from build123d import *

# Parameters (mm, degrees)
BOSS_EXTRUDE1_DEPTH = 3
SKETCH2_W           = 54
SKETCH2_H           = 8
BOSS_EXTRUDE2_DEPTH = 57
SKETCH3_R           = 2.05
CUT_EXTRUDE1_DEPTH  = 57
BOSS_EXTRUDE3_DEPTH = 57
FILLET1_R           = 3
CUT_EXTRUDE2_DEPTH  = 6
FILLET2_R           = 1
FILLET3_R           = 0.8
CHAMFER1_SIZE       = 0.8
CHAMFER2_SIZE       = 0.7


with BuildPart() as part:
    # Sketch1 → Boss-Extrude1 (new body)
    with BuildSketch(Plane.XY):
        Polygon((54, 0), (54, 8), (30, 8), (30, 38), (0, 38), (0, 0), align=None)
    extrude(amount=BOSS_EXTRUDE1_DEPTH)

    # Sketch2 → Boss-Extrude2 (add)
    with BuildSketch(Plane(origin=(0, 0, 0), x_dir=(-1, 0, 0), z_dir=(0, 0, -1))):
        with Locations((-27, 4)):
            Rectangle(SKETCH2_W, SKETCH2_H)
    extrude(amount=BOSS_EXTRUDE2_DEPTH)

    # Sketch3 → Cut-Extrude1 (cut)
    with BuildSketch(Plane.XZ):
        with Locations(Location((40, -1.8, 0), (0, 0, 270))):
            Circle(SKETCH3_R)
        with Locations(Location((40, -50.3, 0), (0, 0, 270))):
            Circle(SKETCH3_R)
    extrude(amount=-CUT_EXTRUDE1_DEPTH, mode=Mode.SUBTRACT)

    # Sketch4 → Boss-Extrude3 (add)
    with BuildSketch(Plane(origin=(0, 0, 0), x_dir=(-1, 0, 0), z_dir=(0, 0, -1))):
        Polygon((-18, 8), (-18, 11), (-23, 11), (-23, 12.85), (-18.25, 17.6), (-11.75, 17.6), (-7, 12.85), (-7, 11), (-12, 11), (-12, 8), align=None)
    extrude(amount=BOSS_EXTRUDE3_DEPTH)

    # Fillet1
    fillet1_edges = [part.edges().sort_by_distance(p)[0] for p in [
        (0, 38, 1.5),
        (30, 38, 1.5),
    ]]
    fillet(fillet1_edges, radius=FILLET1_R)

    # Sketch5 → Cut-Extrude2 (cut)
    with BuildSketch(Plane.XY.offset(3)):
        with BuildLine():
            Line((27.915844453, 26.05), (30, 26.05))
            Line((30, 26.05), (30, 19.95))
            Line((30, 19.95), (27.915844453, 19.95))
            ThreePointArc((27.915844453, 19.95), (27.100066936, 19.836954631), (26.345769332, 19.506338028))
            ThreePointArc((26.345769332, 19.506338028), (20.1, 23), (26.345769332, 26.493661972))
            ThreePointArc((26.345769332, 26.493661972), (27.100066936, 26.163045369), (27.915844453, 26.05))
        make_face()
    extrude(amount=-CUT_EXTRUDE2_DEPTH, mode=Mode.SUBTRACT)

    # Fillet2
    fillet2_edges = [part.edges().sort_by_distance(p)[0] for p in [
        (30, 26.05, 1.5),
        (30, 19.95, 1.5),
        (28.957922227, 26.05, 3),
        (27.100066936, 26.163045369, 3),
        (20.1, 23, 3),
        (27.100066936, 19.836954631, 3),
        (28.957922227, 19.95, 3),
    ]]
    fillet(fillet2_edges, radius=FILLET2_R)

    # Fillet3
    fillet3_edges = [part.edges().sort_by_distance(p)[0] for p in [
        (7, 11, -28.5),
        (7, 12.85, -28.5),
        (11.75, 17.6, -28.5),
        (18.25, 17.6, -28.5),
        (23, 12.85, -28.5),
        (23, 11, -28.5),
    ]]
    fillet(fillet3_edges, radius=FILLET3_R)

    # Chamfer1
    chamfer1_edges = [part.edges().sort_by_distance(p)[0] for p in [
        (20.1, 11, -57),
        (23, 12.159314575, -57),
        (7, 12.159314575, -57),
        (9.375, 15.225, -57),
        (15, 17.6, -57),
        (20.625, 15.225, -57),
        (22.939103626, 12.824775896, -57),
        (18.224775896, 17.539103626, -57),
        (11.775224104, 17.539103626, -57),
        (7.060896374, 12.824775896, -57),
        (7.234314575, 11.234314575, -57),
        (22.765685425, 11.234314575, -57),
        (12, 9.5, -57),
        (9.9, 11, -57),
        (18, 9.5, -57),
    ]]
    chamfer(chamfer1_edges, length=CHAMFER1_SIZE)

    # Chamfer2
    chamfer2_edges = [part.edges().sort_by_distance(p)[0] for p in [
        (40, 8, -48.25),
        (40, 0, -48.25),
        (40, 8, 0.25),
        (40, 0, 0.25),
    ]]
    chamfer(chamfer2_edges, length=CHAMFER2_SIZE)


solid = part.part
Read the model definition and answer for the solid it produces. Units are mm, in the model's axes. A direction names the side the tool comes from. Give positions to 0.01 mm unless a question says otherwise; leave off trailing zeros. Loops run counter-clockwise (first coordinate to the right, second up) from the corner with the lowest first, then second, coordinate; pieces in that order, holes last. Notation, with made-up numbers: (76, 79) -> (127, 79) arc R11 ccw to (127, 83) -> close; hole circle Ø2 at (15, -18). An arc over 180 degrees is marked (long way). Use a Markdown table: item, result.
Q1. Each of these flat-tipped pins is pushed along its axis until it touches: pin 1 (0.6 mm diameter, centred on y = 12, z = -27.5, fed in from +X); pin 2 (1.8 mm diameter, centred on x = 14, z = -36.5, fed in from +Y); pin 3 (0.6 mm diameter, centred on y = 12.5, z = -38.5, fed in from -X). Where does it stop, or does it pass through?
Solved:
| item | result |
|---|---|
| pin 1 | stops at x = 23 |
| pin 2 | stops at y = 17.6 |
| pin 3 | stops at x = 7 |
Q2. Section B-B, the plane z = -1.8 is taken. Determine the outline of the cut face in (x, y), then the cut area to 3 significant figures.
Solved:
| item | result |
|---|---|
| outline | (0, 0) -> (37.25, 0) -> (37.95, 0.7) -> (37.95, 7.3) -> (37.25, 8) -> (18, 8) -> (18, 11) -> (22.2, 11) arc R0.8 ccw to (23, 11.8) -> (23, 12.52) arc R0.8 ccw to (22.77, 13.08) -> (18.48, 17.37) arc R0.8 ccw to (17.92, 17.6) -> (12.08, 17.6) arc R0.8 ccw to (11.52, 17.37) -> (7.23, 13.08) arc R0.8 ccw to (7, 12.52) -> (7, 11.8) arc R0.8 ccw to (7.8, 11) -> (12, 11) -> (12, 8) -> (0, 8) -> close; (42.05, 0.7) -> (42.75, 0) -> (54, 0) -> (54, 8) -> (42.75, 8) -> (42.05, 7.3) -> close |
| area | 499 mm^2 |
Q3. Find the intervals of material crossed by line 1 along Y through (x, z) = (11.5, -52.5); line 2 along X through (y, z) = (9.5, -46.5); line 3 along Y through (x, z) = (19, -42), in increasing order.
Solved:
| item | result |
|---|---|
| line 1 | y = 0 to 8, 11 to 17.35 |
| line 2 | x = 12 to 18 |
| line 3 | y = 0 to 8, 11 to 16.85 |
Q4. Determine the mould class of faces 1 (the face through (27, 5, -57)), 2 (the face through (12, 10, -28)), 3 (the face through (20.368, 14.908, -56.606)) for opening direction Y: pulls with the +Y half, pulls with the -Y half, needs draft (parallel to the pull), parting line crosses it, or undercut.
Solved:
| item | result |
|---|---|
| face 1 | needs draft |
| face 2 | undercut |
| face 3 | pulls with the +Y half |
Q5. A tool of negligible diameter and unlimited length cuts with its end or side. For faces 4 (the face through (18, 9, -28)), 5 (the face through (20.65, 15.2, -27.71)), 6 (the face through (15, 17.6, -28)), 7 (the face through (30, 31, 1)), 8 (the face through (6, 8, -28)), from which of +Z, -Z, +X, -X, +Y, -Y can it reach the whole face along a straight path? Write none if from no direction.
Solved:
| item | result |
|---|---|
| face 4 | -Z, +X |
| face 5 | -Z, +X, +Y |
| face 6 | -Z, +X, -X, +Y |
| face 7 | +Z, -Z, +X, +Y |
| face 8 | -Z, -X |
Q6. Section A-A, the plane x = 40 is taken. Determine the outline of the cut face in (y, z).
Solved:
| item | result |
|---|---|
| outline | (0, -57) -> (8, -57) -> (8, -53.05) -> (7.3, -52.35) -> (0.7, -52.35) -> (0, -53.05) -> close; (0, -47.55) -> (0.7, -48.25) -> (7.3, -48.25) -> (8, -47.55) -> (8, -4.55) -> (7.3, -3.85) -> (0.7, -3.85) -> (0, -4.55) -> close; (0, 0.95) -> (0.7, 0.25) -> (7.3, 0.25) -> (8, 0.95) -> (8, 3) -> (0, 3) -> close |
Q7. Section D-D, the plane z = -25.5 is taken. Determine the outline of the cut face in (x, y).
Solved:
| item | result |
|---|---|
| outline | (0, 0) -> (54, 0) -> (54, 8) -> (18, 8) -> (18, 11) -> (22.2, 11) arc R0.8 ccw to (23, 11.8) -> (23, 12.52) arc R0.8 ccw to (22.77, 13.08) -> (18.48, 17.37) arc R0.8 ccw to (17.92, 17.6) -> (12.08, 17.6) arc R0.8 ccw to (11.52, 17.37) -> (7.23, 13.08) arc R0.8 ccw to (7, 12.52) -> (7, 11.8) arc R0.8 ccw to (7.8, 11) -> (12, 11) -> (12, 8) -> (0, 8) -> close |
Q8. Section C-C, the plane y = 23 is taken. Determine the outline of the cut face in (x, z).
Solved:
| item | result |
|---|---|
| outline | (0, 0) -> (20.1, 0) -> (20.1, 2) arc R1 ccw to (19.1, 3) -> (0, 3) -> close |
